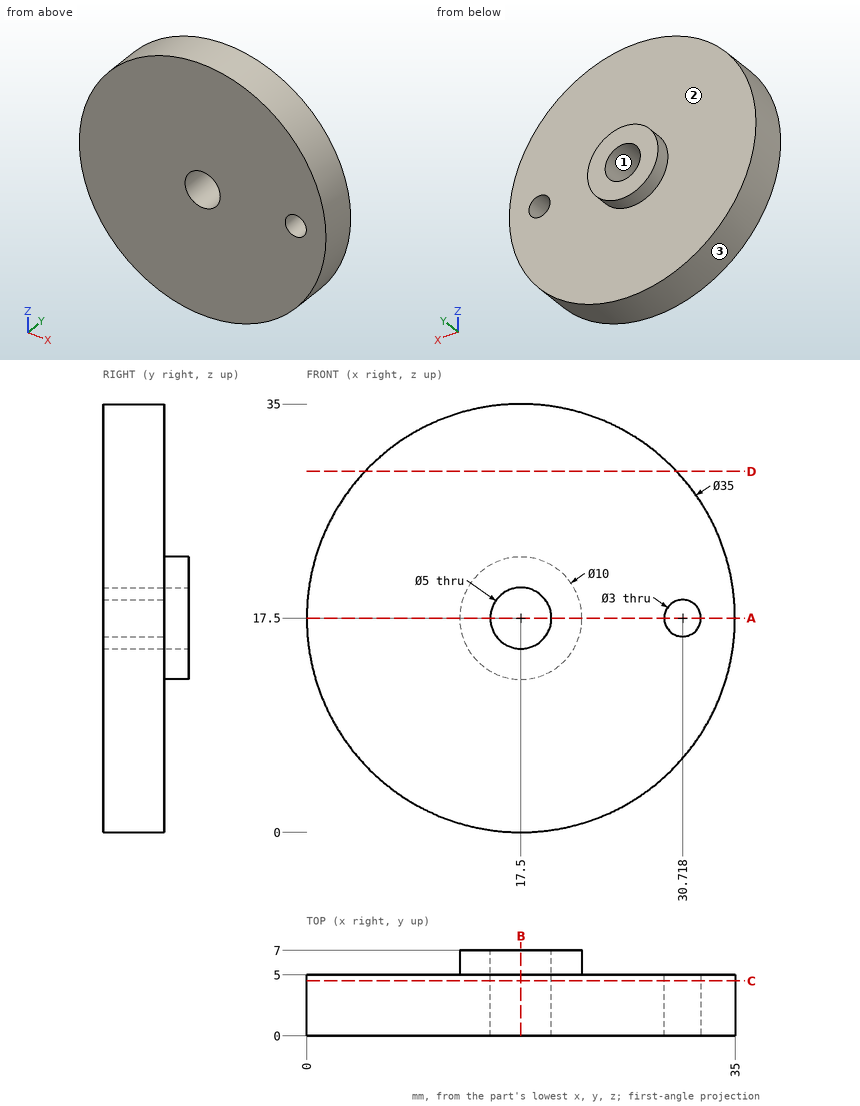
The drawing under review shows one solid part. Ordinate dimensions are in mm from its lowest x, y, z. Coordinates: 2 decimals unless noted, no trailing zeros. Order: outer loops, then holes, each group sorted by start corner. A loop starts at its lowest first (then second) coordinate and runs counter-clockwise, first axis right, second up. Notation, with made-up numbers: (30, 30) -> (87, 30) arc R18 cw to (87, 57) -> close; hole circle Ø7 at (39, -30). An arc over 180 degrees is marked (long way). One line per item, written item: value.
1) We need section C-C, the plane y = 4.5. Give the boundary of the cut face in (x, z), then the cut area to 3 significant figures.
Output values:
outline: circle Ø35 at (17.5, 17.5); hole circle Ø5 at (17.5, 17.5); hole circle Ø3 at (30.72, 17.5)
area: 935 mm2
2) We need section B-B, the plane x = 17.5. Give the boundary of the cut face in (y, z).
Output values:
outline: (0, 0) -> (5, 0) -> (5, 12.5) -> (7, 12.5) -> (7, 15) -> (0, 15) -> close; (0, 20) -> (7, 20) -> (7, 22.5) -> (5, 22.5) -> (5, 35) -> (0, 35) -> close
3) To check wall thickness, follow probe 1 along Z at (x, y) = (17.5, 3.25); probe 2 along Z at (x, y) = (17.5, 5.75); probe 3 along Y at (x, z) = (6, 27). State the ranges of each line that lie inside material, in increasing order. Write a range as [from, to].
Output values:
probe 1: z = [0, 15], [20, 35]
probe 2: z = [12.5, 15], [20, 22.5]
probe 3: y = [0, 5]
4) We need section A-A, the plane z = 17.5. Give the boundary of the cut face in (x, y).
Output values:
outline: (0, 0) -> (15, 0) -> (15, 7) -> (12.5, 7) -> (12.5, 5) -> (0, 5) -> close; (20, 0) -> (29.22, 0) -> (29.22, 5) -> (22.5, 5) -> (22.5, 7) -> (20, 7) -> close; (32.22, 0) -> (35, 0) -> (35, 5) -> (32.22, 5) -> close
5) Clearance check with flat-ended pins moving along their axes: P1, Ø5, axis at x = 9.5, z = 24, coming from the +Y side; P2, Ø1.5, axis at x = 20, z = 20, coming from the -Y side; P3, Ø2, axis at x = 4, y = 4, coming from the +Z side. State where each tip first meets the part, or that it passes through.
Output values:
P1: stops at y = 5
P2: stops at y = 0
P3: stops at z = 29.75
6) We need section D-D, the plane z = 29.5. Give the boundary of the cut face in (x, y).
Output values:
outline: (4.76, 0) -> (30.24, 0) -> (30.24, 5) -> (4.76, 5) -> close
7) Draft analysis for pull direction Z (two halves, no side actions). For the marked faces 1, 2 and 3, state which applies: +Z half, -Z half, draft (parallel to the pull), parting line (faces both ways), or undercut.
Output values:
face 1: undercut
face 2: draft
face 3: parting line
